The listing builds one solid part. Answer for the finished solid, in the listing's coordinates (mm). Give positions to 0.01 mm unless a question says otherwise; leave off trailing zeros. Loops run counter-clockwise (first coordinate to the right, second up) from the corner with the lowest first, then second, coordinate; pieces in that order, holes last. Notation, with made-up numbers: (18.25, -8.5) - (71.25, -8.5) arc R20 ccw to (71.25, 4.5) - close; hole circle Ø11 at (-18.5, -15.5). An arc over 180 degrees is marked (long way). Write item = value, one per line. Start each with the question number.
1) The part is cut by section A-A on z = 280.67. Write down the section's boundary in (x, y) (3 decimals).
2) The part is cut by section C-C on y = -8.5. Write down the section's boundary in (x, z).
3) Flat-ended cylindrical pins translate along their axes: P1, Ø4, axis at x = -35, y = -3, coming from the -Z side; P2, Ø4, axis at x = 13, y = 1, coming from the -Z side. Find the tip coordinate at first contact, or state that the pin passes through.
4) The part is cut by section B-B on x = 16.51. Write down the section's boundary in (y, z) (3 decimals).
5) Consider probe 1 along Z at (x, y) = (16, 9); probe 2 along X at (y, z) = (13, 49); probe 3 along Y at (x, z) = (-9, 35.5). Determine where each line is inside the solid, lowest interval first.
6) The part is cut by section D-D on x = 35. Write down the section's boundary in (y, z), plus the area to 3 significant figures.
from build123d import *

# Parameters (mm, degrees)
SKETCH1_W           = 88.9
SKETCH1_H           = 38.1
BOSS_EXTRUDE1_DEPTH = 330.2
FILLET1_R           = 2.54
CUT_EXTRUDE1_DEPTH  = 406.4
SKETCH3_R           = 3.175
CUT_EXTRUDE2_DEPTH  = 12.7


with BuildPart() as part:
    # Sketch1 → Boss-Extrude1 (new body)
    with BuildSketch(Plane.XY):
        Rectangle(SKETCH1_W, SKETCH1_H)
    extrude(amount=BOSS_EXTRUDE1_DEPTH)

    # Fillet1
    fillet1_edges = [part.edges().sort_by_distance(p)[0] for p in [
        (44.45, -19.05, 165.1),
        (-44.45, -19.05, 165.1),
        (-44.45, 19.05, 165.1),
        (44.45, 19.05, 165.1),
    ]]
    fillet(fillet1_edges, radius=FILLET1_R)

    # Sketch2 → Cut-Extrude1 (cut)
    with BuildSketch(Plane.ZY.offset(44.45)):
        Polygon((0, 19.05), (0, -19.05), (38.1, 19.05), align=None)
    cut_extrude1 = extrude(amount=-CUT_EXTRUDE1_DEPTH, mode=Mode.SUBTRACT)

    # Mirror1: Cut-Extrude1 across plane
    add(cut_extrude1.mirror(Plane.XY.offset(165.1)), mode=Mode.SUBTRACT)

    # Sketch3 → Cut-Extrude2 (cut)
    with BuildSketch(Plane(origin=(0, 19.05, 0), x_dir=(1, 0, 0), z_dir=(0, 1, 0))):
        with Locations((16.51, -49.53)):
            Circle(SKETCH3_R)
    cut_extrude2 = extrude(amount=-CUT_EXTRUDE2_DEPTH, mode=Mode.SUBTRACT)

    # Mirror2: Cut-Extrude2 across plane
    add(cut_extrude2.mirror(Plane.XY.offset(165.1)), mode=Mode.SUBTRACT)


solid = part.part
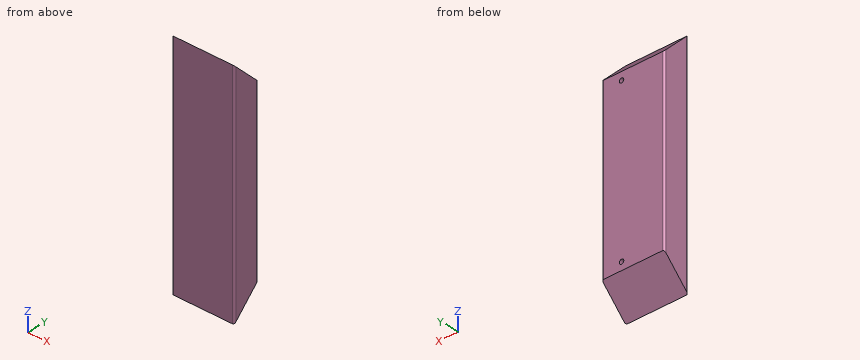
Answer below:
q1.outline = (-44.45, -16.51) arc R2.54 ccw to (-41.91, -19.05) - (41.91, -19.05) arc R2.54 ccw to (44.45, -16.51) - (44.45, 16.51) arc R2.54 ccw to (41.91, 19.05) - (19.685, 19.05) - (19.685, 6.35) - (13.335, 6.35) - (13.335, 19.05) - (-41.91, 19.05) arc R2.54 ccw to (-44.45, 16.51) - close
q2.outline = (-44.45, 10.55) - (44.45, 10.55) - (44.45, 319.65) - (-44.45, 319.65) - close
q3.P1 = 14.05
q3.P2 = 18.05
q4.outline = (-19.05, 0) - (19.05, 38.1) - (19.05, 46.355) - (6.35, 46.355) - (6.35, 52.705) - (19.05, 52.705) - (19.05, 277.495) - (6.35, 277.495) - (6.35, 283.845) - (19.05, 283.845) - (19.05, 292.1) - (-19.05, 330.2) - close
q5.probe_1 = 28.05 to 46.4, 52.66 to 277.54, 283.8 to 302.15
q5.probe_2 = -44.45 to 13.38, 19.64 to 44.45
q5.probe_3 = -19.05 to 16.45
q6.outline = (-19.05, 0) - (19.05, 38.1) - (19.05, 292.1) - (-19.05, 330.2) - close
q6.area = 11,100 mm2
